Source: three-view drawing plus pictorial views. Frame: mm from the lowest corner of the part. Give positions to 0.01 mm unless a question says otherwise; leave off trailing zeros. Order: outer loops, then holes, each group sorted by start corner. A loop starts at its lowest first (then second) coordinate and runs counter-clockwise, first axis right, second up. Notation, with made-up numbers: M 34,10 L 83,10 A19 cw 83,30 Z; hole C -19.75,-29 d3. An arc over 180 degrees is marked long. Use CSV: the item, a comma, the result in double quotes. Start each with the question number.
Item 1: Section query D-D on y = 10.5. Return loops of the section in (x, z).
Item 2: Section query B-B on z = 15.9. Return loops of the section in (x, y), and give its area (3 significant figures).
Item 3: First-contact query: pin 1 (6 mm diameter, centred on x = 6.5, y = 3.5, fed in from -Z); pin 2 (1.6 mm diameter, centred on y = 7, z = 1.5, fed in from -X); pin 3 (4 mm diameter, centred on x = 25, z = 8.5, fed in from -Y); pin 4 (3 mm diameter, centred on y = 10.5, z = 18, fed in from -X). Flat tips, straight axial feed; report the tip coordinate or a pass-through.
Item 4: Section query C-C on y = 2. Return loops of the section in (x, z).
Item 5: Section query A-A on x = 15.9. Return loops of the section in (y, z), and give its area (3 significant figures).
Item 6: Ray query, probe 1 along Z at (x, y) = (15.9, 16.25); probe 2 along Z at (x, y) = (11, 4). Return the intervals inside material, ascending. Write a range as from..to.
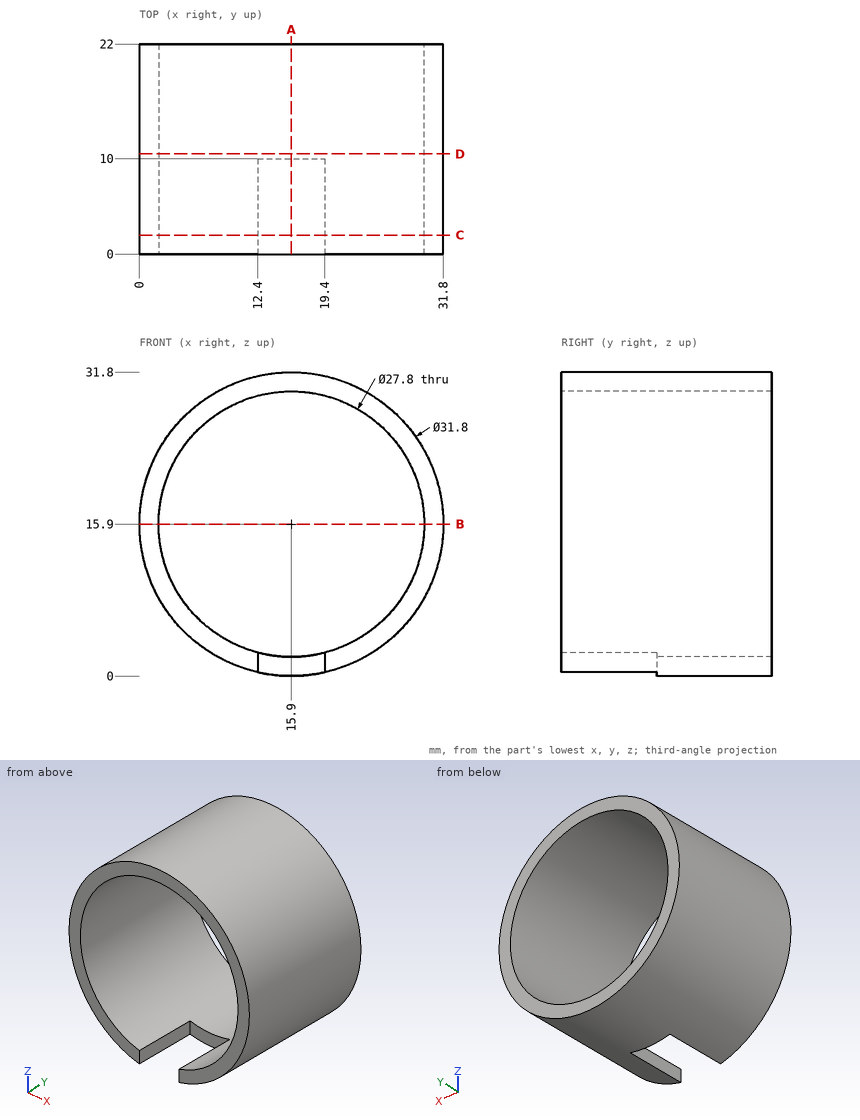
Verdict:
1,outline,"C 15.9,15.9 d31.8; hole C 15.9,15.9 d27.8"
2,outline,"M 0,0 L 2,0 L 2,22 L 0,22 Z; M 29.8,0 L 31.8,0 L 31.8,22 L 29.8,22 Z"
2,area,"88.0 mm2"
3,pin 1,"z = 1.34"
3,pin 2,"x = 7.66"
3,pin 3,"through"
3,pin 4,"x = 0.01"
4,outline,"M 12.4,0.39 L 12.4,2.45 A13.9 cw long 19.4,2.45 L 19.4,0.39 A15.9 ccw long Z"
5,outline,"M 0,29.8 L 22,29.8 L 22,31.8 L 0,31.8 Z; M 10,0 L 22,0 L 22,2 L 10,2 Z"
5,area,"68.0 mm2"
6,probe 1,"0..2, 29.8..31.8"
6,probe 2,"0.77..2.89, 28.91..31.03"
